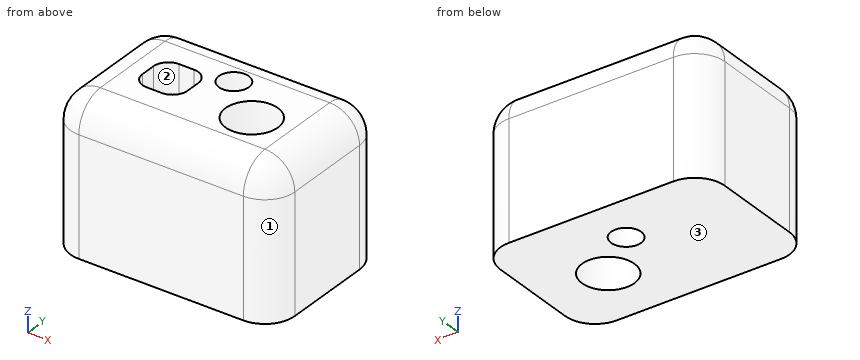
```python
from build123d import *

# Parameters (mm, degrees)
F0_W     = 60
F0_H     = 40
F1_DEPTH = 39.5
F2_R     = 8
F3_W     = 12
F3_H     = 12
F4_DEPTH = 15
F5_R     = 4
F6_R     = 4
F6_R_2   = 7
F7_DEPTH = 39.501


with BuildPart() as f1:
    # F0 (on Top) → F1 (new body)
    with BuildSketch(Plane.XY):
        with Locations((30, 20)):
            Rectangle(F0_W, F0_H)
    extrude(amount=F1_DEPTH)

    # F2
    f2_edges = [f1.edges().sort_by_distance(p)[0] for p in [
        (0, 20, 39.5),
        (30, 0, 39.5),
        (60, 20, 39.5),
        (30, 40, 39.5),
        (60, 0, 19.75),
        (60, 40, 19.75),
        (0, 0, 19.75),
        (0, 40, 19.75),
    ]]
    fillet(f2_edges, radius=F2_R)

    # F3 (on face) → F4 (cut)
    with BuildSketch(Plane.XY.offset(39.5)):
        with Locations((18.08178, 20)):
            Rectangle(F3_W, F3_H)
    extrude(amount=-F4_DEPTH, mode=Mode.SUBTRACT)

    # F5
    f5_edges = [f1.edges().sort_by_distance(p)[0] for p in [
        (12.08178, 26, 32),
        (12.08178, 14, 32),
        (24.08178, 26, 32),
        (24.08178, 14, 32),
    ]]
    fillet(f5_edges, radius=F5_R)

    # F6 (on face) → F7 (cut, through all)
    with BuildSketch(Plane.XY.offset(39.5)):
        with Locations((30, 27)):
            Circle(F6_R)
        with Locations((42, 17)):
            Circle(F6_R_2)
    extrude(amount=-F7_DEPTH, mode=Mode.SUBTRACT)


solid = f1.part
```
Input: part model. Units: mm. Frame: model coordinates. Face numbers are marked on the shaded views. Coordinates: 2 decimals unless noted, no trailing zeros. Loops run counter-clockwise (first coordinate to the right, second up) from the corner with the lowest first, then second, coordinate; pieces in that order, holes last. Notation, with made-up numbers: M 22,-6 L 50,-6 A21 cw 50,33 Z; hole C 45,-16.75 d3. An arc over 180 degrees is marked long. Use a Markdown table: item, result. Add a question column.
1) Section A-A, the plane y = 27. Return the cut outline in (x, z).
2) Draft query along Y for the marked faces 1, 2 and 3. Return one class per face: +Y half, -Y half, draft (parallel to the pull), parting line (faces both ways), or undercut.
3) Section D-D, the plane z = 12. Return the cut outline in (x, y), plus the area to 3 significant figures.
4) Pin query (flat end, axial travel): P1, Ø2, axis at x = 17.5, z = 33, coming from the +Y side; P2, Ø6, axis at x = 20, y = 20.5, coming from the +Z side; P3, Ø1, axis at y = 4.5, z = 30.5, coming from the -X side. Return the tip coordinate at first contact, or that it passes through.
5) Section B-B, the plane x = 42. Return the cut outline in (y, z).
6) Section C-C, the plane z = 29. Return the cut outline in (x, y), plus the area to 3 significant figures.
7) Line query: L1, parallel to Y at x = 42, z = 9.5; L2, parallel to Y at x = 30, z = 28; L3, parallel to X at y = 15.5, z = 28.5. Output: solid intervals per line, ascending. Write a range as from..to.
Answer below:
| question | item | result |
|---|---|---|
| 1 | outline | M 0,0 L 26,0 L 26,39.5 L 8,39.5 A8 ccw 0,31.5 Z; M 34,0 L 60,0 L 60,31.5 A8 ccw 52,39.5 L 34,39.5 Z |
| 2 | face 1 | -Y half |
| 2 | face 2 | undercut |
| 2 | face 3 | draft |
| 3 | outline | M 0,8 A8 ccw 8,0 L 52,0 A8 ccw 60,8 L 60,32 A8 ccw 52,40 L 8,40 A8 ccw 0,32 Z; hole C 30,27 d8; hole C 42,17 d14 |
| 3 | area | 2,140 mm2 |
| 4 | P1 | y = 39.98 |
| 4 | P2 | z = 24.5 |
| 4 | P3 | x = 0.58 |
| 5 | outline | M 0,0 L 10,0 L 10,39.5 L 8,39.5 A8 ccw 0,31.5 Z; M 24,0 L 40,0 L 40,31.5 A8 ccw 32,39.5 L 24,39.5 Z |
| 6 | outline | M 0,8 A8 ccw 8,0 L 52,0 A8 ccw 60,8 L 60,32 A8 ccw 52,40 L 8,40 A8 ccw 0,32 Z; hole M 12.08,18 A4 ccw 16.08,14 L 20.08,14 A4 ccw 24.08,18 L 24.08,22 A4 ccw 20.08,26 L 16.08,26 A4 ccw 12.08,22 Z; hole C 30,27 d8; hole C 42,17 d14 |
| 6 | area | 2,010 mm2 |
| 7 | L1 | 0..10, 24..40 |
| 7 | L2 | 0..23, 31..40 |
| 7 | L3 | 0..12.96, 23.2..35.16, 48.84..60 |
